Check sheet for the drawn part. Datum: minimum x, y, z corner. Units: mm. A direction names the side the tool comes from. Round coordinates to 2 decimals unless told otherwise and drop trailing zeros. Write each loop counter-clockwise with the first axis right and the second up, starting at its lowest first coordinate (ties: lowest second). Pieces come first, ordered by that corner, then holes. Notation, with made-up numbers: (7.5, 58) - (14.5, 58) arc R28 cw to (14.5, 87) - close; hole circle Ø3 at (-20.75, 41.25). An arc over 180 degrees is marked (long way). Answer as a JSON object with one key per item and string values. Group by question number.
1) Set-up check for the marked faces 4, 5 and 6: record each of +Z, -Z, +X, -X, +Y, -Y from which the full face is reachable in a straight line by a thin tool's end or side.
2) Mould release check, pull along Z, two halves, no side actions. Record for the marked faces 1, 2 and 3: +Z half, -Z half, draft (parallel to the pull), parting line (faces both ways), or undercut.
3) Go/stop test with flat-tipped pins: pin 1 Ø1 at (y, z) = (43, 16) entering from -X; pin 2 Ø3 at (x, z) = (38, 2) entering from -Y; pin 3 Ø1.5 at (y, z) = (50.5, 5) entering from -X; pin 4 Ø6.5 at (y, z) = (40.5, 2.5) entering from +X. Record where each tip stops, or that it passes through.
4) Thickness scan on line 1 (Y direction, x = 16, z = 6.6); line 2 (X direction, y = 68, z = 6.6); line 3 (Y direction, x = 20.5, z = 11.25). Record the ranges inside material, lowest first.
5) Section check C-C (y = 68). Enter the section's corners in (x, z).
6) Section check D-D (x = 16). Enter the section's corners in (y, z).
7) Section check B-B (z = 9.5). Enter the section's corners in (x, y).
8) Section check A-A (x = 62). Enter the section's corners in (y, z), then the cut area to 3 significant figures.
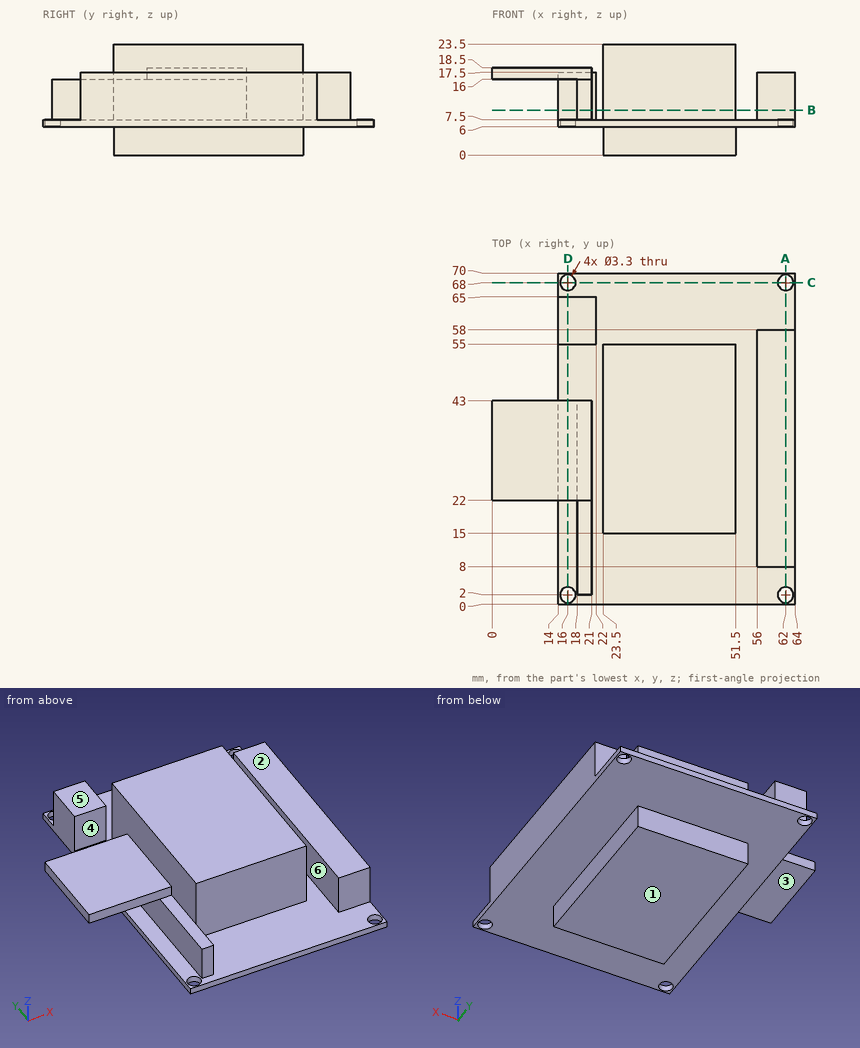
Returned:
{
 "1": {"face 4": "+Z, -X", "face 5": "+Z, +X, -X, +Y", "face 6": "+Z, +Y, -Y"},
 "2": {"face 1": "-Z half", "face 2": "+Z half", "face 3": "undercut"},
 "3": {"pin 1": "x = 0", "pin 2": "y = 15", "pin 3": "x = 23.5", "pin 4": "x = 51.5"},
 "4": {"line 1": "0 to 0.35, 3.65 to 66.35, 69.65 to 70", "line 2": "14 to 14.35, 17.65 to 60.35, 63.65 to 64", "line 3": "2 to 43, 55 to 65"},
 "5": {"outline": "(14, 6) - (14.35, 6) - (14.35, 7.5) - (14, 7.5) - close; (17.65, 6) - (60.35, 6) - (60.35, 7.5) - (17.65, 7.5) - close; (63.65, 6) - (64, 6) - (64, 7.5) - (63.65, 7.5) - close"},
 "6": {"outline": "(0, 6) - (0.35, 6) - (0.35, 7.5) - (0, 7.5) - close; (3.65, 6) - (66.35, 6) - (66.35, 7.5) - (65, 7.5) - (65, 17.5) - (55, 17.5) - (55, 7.5) - (3.65, 7.5) - close; (22, 16) - (43, 16) - (43, 18.5) - (22, 18.5) - close; (69.65, 6) - (70, 6) - (70, 7.5) - (69.65, 7.5) - close"},
 "7": {"outline": "(14, 55) - (22, 55) - (22, 65) - (14, 65) - close; (18, 2) - (21, 2) - (21, 43) - (18, 43) - close; (23.5, 15) - (51.5, 15) - (51.5, 55) - (23.5, 55) - close; (56, 8) - (64, 8) - (64, 58) - (56, 58) - close"},
 "8": {"outline": "(0, 6) - (0.35, 6) - (0.35, 7.5) - (0, 7.5) - close; (3.65, 6) - (66.35, 6) - (66.35, 7.5) - (58, 7.5) - (58, 17.5) - (8, 17.5) - (8, 7.5) - (3.65, 7.5) - close; (69.65, 6) - (70, 6) - (70, 7.5) - (69.65, 7.5) - close", "area": "595 mm2"}
}
